Here's the drawing with two shaded views (mm, measured from the low corner). I have some questions. A direction names the side the tool comes from. Coordinates: 2 decimals unless noted, no trailing zeros. Loops run counter-clockwise (first coordinate to the right, second up) from the corner with the lowest first, then second, coordinate; pieces in that order, holes last. Notation, with made-up numbers: (37.25, -40) - (50.25, -40) arc R21 ccw to (50.25, -31) - close; hole circle Ø5 at (16.25, 36). An arc over 180 degrees is marked (long way). One line per item, written item: value. Start each with the question number.
(1) I'm going to push flat-ended pins straight in: P1, Ø2, axis at y = 27.5, z = 5, coming from the -X side; P2, Ø2, axis at x = 37.64, y = 26.41, coming from the -Z side; P3, Ø4.5, axis at x = 21, y = 3.5, coming from the -Z side; P4, Ø1, axis at y = 11, z = 3, coming from the +X side. Where does each tip first touch, or does it pass through?
(2) If I drill on line 1 along X through (y, z) = (26.5, 4) (1 decimal); line 2 along X through (y, z) = (36, 5.4) (1 decimal); line 3 along X through (y, z) = (14, 3.75) (1 decimal), over which ranges is the centre line in solid material (lowest first)? Write a range as from..to.
(3) If we section it at A-A on y = 21: Write out the boundary of the cut face in (x, z).
(4) If we mould it in two halves opening along Y, with no side actions, what happens to the marked faces 1, 2 and 3? For each: pulls with the +Y half, pulls with the -Y half, needs draft (parallel to the pull), parting line crosses it, or undercut.
(5) On a 3-axis mill with a long thin cutter (end or side, diameter ignored), from which of +Z, -Z, +X, -X, +Y, -Y can I reach the whole of each face in a straight line? I mean the marked faces 4 and 5. Say none if no direction works.
(6) If we section it at B-B on x = 38: Write out the boundary of the cut face in (y, z).
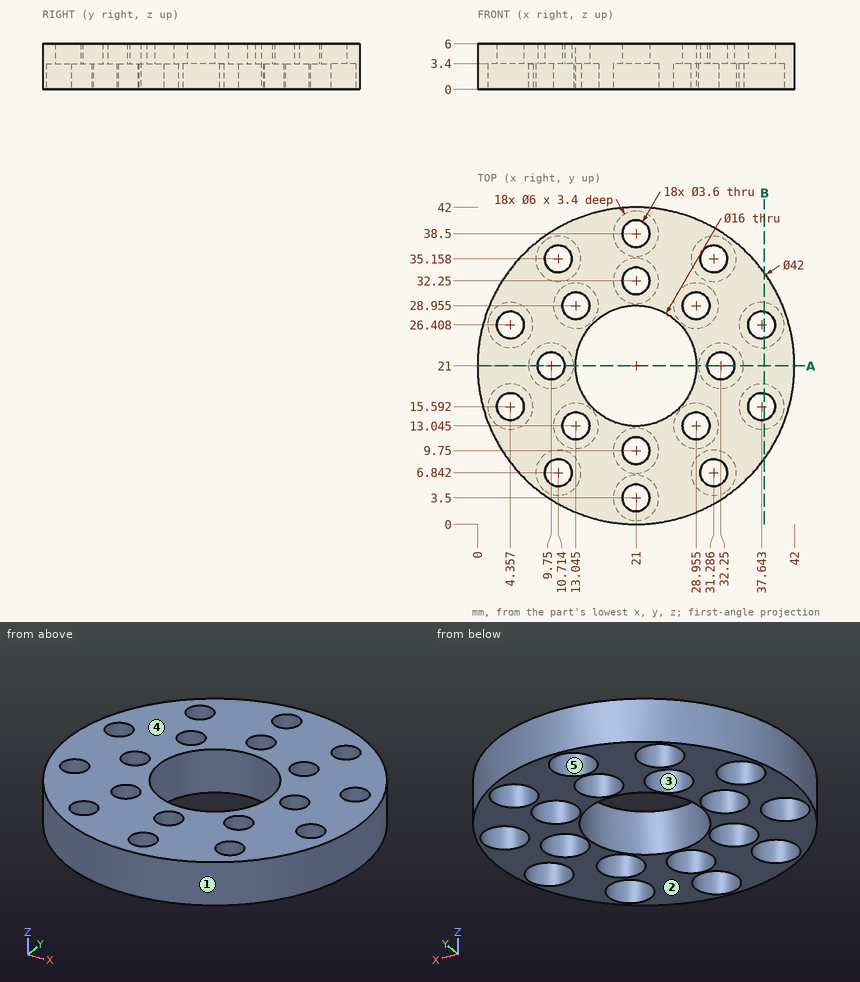
Values:
1. P1: stops at x = 0.73
1. P2: passes through
1. P3: stops at z = 3.4
1. P4: stops at x = 39.73
2. line 1: x = 0.7..2.6, 6.2..15.2, 26.8..35.8, 39.4..41.3
2. line 2: x = 6.3..9.1, 12.3..29.7, 32.9..35.7
2. line 3: x = 1.2..3.5, 5.2..11.5, 14.6..17.1, 24.9..27.4, 30.5..36.8, 38.5..40.8
3. outline: (0, 0) - (6.75, 0) - (6.75, 3.4) - (7.95, 3.4) - (7.95, 6) - (0, 6) - close; (11.55, 3.4) - (12.75, 3.4) - (12.75, 0) - (13, 0) - (13, 6) - (11.55, 6) - close; (29, 0) - (29.25, 0) - (29.25, 3.4) - (30.45, 3.4) - (30.45, 6) - (29, 6) - close; (34.05, 3.4) - (35.25, 3.4) - (35.25, 0) - (42, 0) - (42, 6) - (34.05, 6) - close
4. face 1: parting line crosses it
4. face 2: needs draft
4. face 3: undercut
5. face 4: +Z, +X, -X, +Y, -Y
5. face 5: -Z
6. outline: (8.67, 0) - (12.61, 0) - (12.61, 3.4) - (13.83, 3.4) - (13.83, 6) - (8.67, 6) - close; (17.36, 3.4) - (18.57, 3.4) - (18.57, 0) - (23.43, 0) - (23.43, 3.4) - (24.64, 3.4) - (24.64, 6) - (17.36, 6) - close; (28.17, 3.4) - (29.39, 3.4) - (29.39, 0) - (33.33, 0) - (33.33, 6) - (28.17, 6) - close
